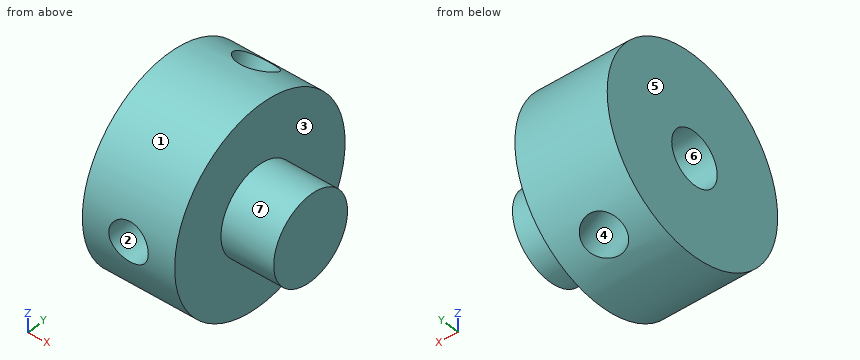
```python
from build123d import *

# Parameters (mm, degrees)
F0_R     = 15.001136
F0_R_2   = 4
F1_DEPTH = 14
F3_R     = 3
F4_DEPTH = 25
F5_COUNT = 3
F7_R     = 6.5
F8_DEPTH = 8


with BuildPart() as f1:
    # F0 (on Right) → F1 (new body)
    with BuildSketch(Plane.YZ):
        with Locations((-77.428193, 78.135299)):
            Circle(F0_R)
        with Locations((-77.781746, 77.781746)):
            Circle(F0_R_2, mode=Mode.SUBTRACT)
    extrude(amount=F1_DEPTH)


with BuildPart() as f4:
    # F3 (on face) → F4 (new body)
    with BuildSketch(Plane.XZ.offset(77.428193)):
        with Locations((7, 78.135299)):
            Circle(F3_R)
    extrude(amount=F4_DEPTH)


with BuildPart() as f5_1:
    # F5: instance of F4
    add(f4.part.rotate(Axis((0, -77.428193, 78.135299), (1, 0, 0)), 1 * 360 / F5_COUNT))


with BuildPart() as f5_2:
    # F5: instance of F4
    add(f4.part.rotate(Axis((0, -77.428193, 78.135299), (1, 0, 0)), 2 * 360 / F5_COUNT))


with BuildPart() as f1_1:
    add(f1.part)

    # F6: cut F4, F5_1, F5_2
    add(f4.part, mode=Mode.SUBTRACT)
    add(f5_1.part, mode=Mode.SUBTRACT)
    add(f5_2.part, mode=Mode.SUBTRACT)

    # F7 (on face) → F8 (join)
    with BuildSketch(Plane.YZ.offset(14)):
        with Locations((-77.781746, 77.781746)):
            Circle(F7_R)
    extrude(amount=F8_DEPTH)


solid = f1_1.part
```
Could you check a few things on this model? Use its own coordinates, in mm. Face numbers are marked on the shaded views. A direction names the side the tool comes from. Give positions to 0.01 mm unless a question says otherwise; leave off trailing zeros. Write each loop counter-clockwise with the first axis right and the second up, starting at its lowest first coordinate (ties: lowest second). Pieces come first, ordered by that corner, then holes. Notation, with made-up numbers: (10.5, -16.75) -> (26.5, -16.75) arc R32 cw to (26.5, 14.25) -> close; hole circle Ø7 at (-13, 65). An arc over 180 degrees is marked (long way). Write each question's results on one line, items separated by ' | '.
1. I want a section at A-A, the plane x = 5.75. Write out the boundary of the cut face in (y, z), then the cut area to 3 significant figures.
Check sheet entries:
outline: (-92.18, 75.41) arc R15 ccw to (-72.41, 64) -> (-78.07, 73.79) arc R4 cw to (-81, 75.41) -> close; (-92.18, 80.86) -> (-80.33, 80.86) arc R4 cw to (-78.51, 81.71) -> (-72.41, 92.27) arc R15 ccw to start; (-73.91, 78.78) arc R4 cw to (-73.81, 77.32) -> (-67.69, 66.72) arc R15 ccw to (-67.69, 89.55) -> close | area: 472 mm²
2. I want a section at D-D, the plane x = 2.5. Write out the boundary of the cut face in (y, z), then the cut area to 3 significant figures.
Check sheet entries:
outline: circle Ø30 at (-77.43, 78.14); hole circle Ø8 at (-77.78, 77.78) | area: 657 mm²
3. I need wall thicknesses on L1, parallel to X at y = -90.5, z = 78; L2, parallel to X at y = -80, z = 70; L3, parallel to Z at x = 19.75, y = -78. Which ranges of each line are inside material? Lowest first, please.
Check sheet entries:
L1: x = 0 to 4, 10 to 14 | L2: x = 0 to 14 | L3: z = 71.29 to 84.28
4. If we mould it in two halves opening along Y, with no side actions, what happens to the marked faces 4, 5, 6 and 7? For each: released by +Y, released by -Y, zero draft, split by the parting line, or undercut.
Check sheet entries:
face 4: undercut | face 5: zero draft | face 6: undercut | face 7: split by the parting line
5. On a 3-axis mill with a long thin cutter (end or side, diameter ignored), from which of +Z, -Z, +X, -X, +Y, -Y can I reach the whole of each face in a straight line? I mean the marked faces 1, 2 and 3. Say none if no direction works.
Check sheet entries:
face 1: +X, -X | face 2: -Y | face 3: +X
6. Will these pins go through, and if not, where does the flat tip stop? pin 1 Ø2 at (x, z) = (2.5, 81) entering from +Y; pin 2 Ø2 at (x, z) = (7, 69.5) entering from -Y; pin 3 Ø6 at (x, z) = (5.5, 89.5) entering from +Y; pin 4 Ø6.5 at (y, z) = (-78, 79) entering from -X.
Check sheet entries:
pin 1: stops at y = -62.54 | pin 2: stops at y = -90.34 | pin 3: stops at y = -64.98 | pin 4: stops at x = 0
7. I want a section at C-C, the plane x = 18. Write out the boundary of the cut face in (y, z).
Check sheet entries:
outline: circle Ø13 at (-77.78, 77.78)
8. I want a section at B-B, the plane y = -85.5. Write out the boundary of the cut face in (x, z), then the cut area to 3 significant figures.
Check sheet entries:
outline: (0, 65.49) -> (14, 65.49) -> (14, 90.78) -> (0, 90.78) -> close; hole circle Ø6 at (7, 78.14) | area: 326 mm²
